```python
from build123d import *

# Parameters (mm, degrees)
SKETCH_1_R      = 0.9
SKETCH_1_W      = 12.938114719
SKETCH_1_H      = 2
EXTRUDE_1_DEPTH = 2


with BuildPart() as part:
    # 草图1 → 凸台-拉伸1 (new body)
    with BuildSketch(Plane.XY):
        with BuildLine():
            Line((42, 1), (45, 1))
            Line((45, 1), (41, 5))
            Line((41, 5), (-24.453286313, 8.983379328))
            ThreePointArc((-24.453286313, 8.983379328), (-24.726516864, 8.995843872), (-25, 9))
            ThreePointArc((-25, 9), (-27.25, 6.75), (-25, 4.5))
            ThreePointArc((-25, 4.5), (-20.5, 0), (-25, -4.5))
            ThreePointArc((-25, -4.5), (-27.25, -6.75), (-25, -9))
            ThreePointArc((-25, -9), (-24.726516864, -8.995843872), (-24.453286313, -8.983379328))
            Line((-24.453286313, -8.983379328), (41, -5))
            Line((41, -5), (45, -1))
            Line((45, -1), (42, -1))
            Line((42, -1), (42, 1))
        make_face()
        with Locations((-25, 6.75)):
            Circle(SKETCH_1_R, mode=Mode.SUBTRACT)
        with Locations((-25, -6.75)):
            Circle(SKETCH_1_R, mode=Mode.SUBTRACT)
        with Locations((-14, 0)):
            Circle(SKETCH_1_R, mode=Mode.SUBTRACT)
        Polygon((5, 1.05), (3.6, 1.05), (3.6, 3.15), (0.5, 3.15), (0.5, 1.05), (-3.5, 1.05), (-3.5, -1.05), (5, -1.05), align=None, mode=Mode.SUBTRACT)
        with Locations((32.530942641, 0)):
            Rectangle(SKETCH_1_W, SKETCH_1_H, mode=Mode.SUBTRACT)
        Polygon((24.030895161, -2.05), (11.162143386, -2.463125002), (9.25663283, -1.05), (7.998759736, -1.05), (7.998759736, 1.05), (9.25663283, 1.05), (11.162143386, 2.463125002), (24.030895161, 2.05), align=None, mode=Mode.SUBTRACT)
    extrude(amount=EXTRUDE_1_DEPTH)


solid = part.part
```
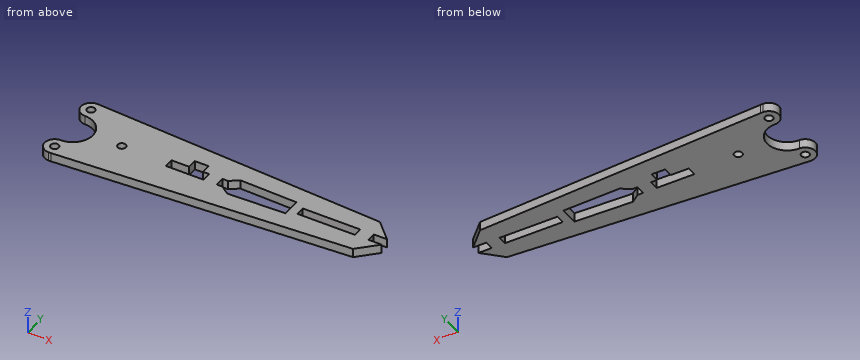
Input: part model. Units: mm. Frame: model coordinates. Round coordinates to 2 decimals unless told otherwise and drop trailing zeros. Loops run counter-clockwise (first coordinate to the right, second up) from the corner with the lowest first, then second, coordinate; pieces in that order, holes last. Notation, with made-up numbers: M 45,68.5 L 100,68.5 A30 cw 100,91.5 Z; hole C -28,5 d3. An arc over 180 degrees is marked long. Answer in a Markdown table with one row per item. Add a question column.
1. Ray query, probe 1 along Y at (x, z) = (-25, 1.4); probe 2 along Y at (x, z) = (-14, 1.3); probe 3 along Y at (x, z) = (33, 1.1). Return the intervals inside material, ascending.
2. Section D-D (z = 1.1). Give the number of separate pieces and of enclosed holes in the cut face, and give its area (3 significant figures).
3. Contact query for flat-ended pins moving along their axis: pin 1 (1 mm diameter, centred on x = -11.5, z = 0.5, fed in from -Y); pin 2 (0.6 mm diameter, centred on y = 0, z = 1.5, fed in from +X); pin 3 (0.6 mm diameter, centred on y = -0.5, z = 1, fed in from -X). Output: stop coordinate, or through.
4. Section C-C (y = 6.75). Output: boundary loops of the cut face in (x, z), and give its area (3 significant figures).
5. Section B-B (x = 31.5). Output: boundary loops of the cut face in (y, z), and give its area (3 significant figures).
6. Section A-A (y = 0). Output: boundary loops of the cut face in (x, z), and give its area (3 significant figures).
Values follow:
| question | item | result |
|---|---|---|
| 1 | probe 1 | -9 to -7.65, -5.85 to -4.5, 4.5 to 5.85, 7.65 to 9 |
| 1 | probe 2 | -8.35 to -0.9, 0.9 to 8.35 |
| 1 | probe 3 | -5.49 to -1, 1 to 5.49 |
| 2 | separate pieces | 1 |
| 2 | enclosed holes | 6 |
| 2 | area | 802 mm^2 |
| 3 | pin 1 | y = -8.23 |
| 3 | pin 2 | x = 42 |
| 3 | pin 3 | x = -20.57 |
| 4 | outline | M -27.25,0 L -25.9,0 L -25.9,2 L -27.25,2 Z; M -24.1,0 L 12.24,0 L 12.24,2 L -24.1,2 Z |
| 4 | area | 75.4 mm^2 |
| 5 | outline | M -5.58,0 L -1,0 L -1,2 L -5.58,2 Z; M 1,0 L 5.58,0 L 5.58,2 L 1,2 Z |
| 5 | area | 18.3 mm^2 |
| 6 | outline | M -20.5,0 L -14.9,0 L -14.9,2 L -20.5,2 Z; M -13.1,0 L -3.5,0 L -3.5,2 L -13.1,2 Z; M 5,0 L 8,0 L 8,2 L 5,2 Z; M 24.03,0 L 26.06,0 L 26.06,2 L 24.03,2 Z; M 39,0 L 42,0 L 42,2 L 39,2 Z |
| 6 | area | 46.5 mm^2 |
